from build123d import *

# Parameters (mm, degrees)
SKETCH2_W               = 19.05
SKETCH2_H               = 6.35
BOSS_EXTRUDE1_DEPTH     = 2.54
SKETCH3_W               = 2.54
SKETCH3_H               = 6.35
BOSS_EXTRUDE2_DEPTH     = 17.78
FILLET1_R               = 6.35
SKETCH4_R               = 1.143
CUT_EXTRUDE1_DEPTH      = 27.820764344
CUT_EXTRUDE2_DEPTH      = 27.940768363
CUT_EXTRUDE2_DEPTH_BACK = 27.940768363
SKETCH5_R               = 1.143


with BuildPart() as part:
    # Sketch2 → Boss-Extrude1 (new body)
    with BuildSketch(Plane(origin=(0, 0, 0), x_dir=(1, 0, 0), z_dir=(0, 1, 0))):
        with Locations((9.525, 3.175)):
            Rectangle(SKETCH2_W, SKETCH2_H)
    extrude(amount=BOSS_EXTRUDE1_DEPTH)

    # Sketch3 → Boss-Extrude2 (add)
    with BuildSketch(Plane(origin=(0, 2.54, 0), x_dir=(1, 0, 0), z_dir=(0, 1, 0))):
        with Locations((17.78, 3.175)):
            Rectangle(SKETCH3_W, SKETCH3_H)
    extrude(amount=BOSS_EXTRUDE2_DEPTH)

    # Fillet1
    fillet1_edges = [part.edges().sort_by_distance(p)[0] for p in [
        (16.51, 2.54, -3.175),
    ]]
    fillet(fillet1_edges, radius=FILLET1_R)

    # Sketch4 → Cut-Extrude1 (cut, through all)
    with BuildSketch(Plane(origin=(0, 2.54, 0), x_dir=(1, 0, 0), z_dir=(0, 1, 0))):
        with Locations(Location((6.35, 3.175, 0), (0, 0, 270))):
            Circle(SKETCH4_R)
    extrude(amount=-CUT_EXTRUDE1_DEPTH, mode=Mode.SUBTRACT)

    # Sketch5 → Cut-Extrude2 (cut, two sides: drawn at the far end of the back side and taken through both)
    with BuildSketch(Plane.ZY.offset(-16.51).offset(-CUT_EXTRUDE2_DEPTH_BACK)):
        with Locations((-3.175, 15.24)):
            Circle(SKETCH5_R)
        with Locations((-3.175, 4.826)):
            Circle(SKETCH5_R)
    extrude(amount=CUT_EXTRUDE2_DEPTH + CUT_EXTRUDE2_DEPTH_BACK, mode=Mode.SUBTRACT)


solid = part.part
Source: CAD feature listing. Evaluate the final solid. Frame: model axes, mm. A direction names the side the tool comes from. Round coordinates to 2 decimals unless told otherwise and drop trailing zeros. Loops run counter-clockwise (first coordinate to the right, second up) from the corner with the lowest first, then second, coordinate; pieces in that order, holes last.
Q1. First-contact query: P1, Ø1, axis at x = 14.5, z = -1, coming from the +Y side; P2, Ø1.8, axis at x = 6.35, z = -3.175, coming from the +Y side; P3, Ø1.9, axis at x = 4, z = -3, coming from the +Y side. Flat tips, straight axial feed; report the tip coordinate or a pass-through.
Q2. Section C-C, the plane z = -2.5. Return loops of the section in (x, y).
Q3. Access query for faces 1 (the face through (5, 2.54, -3)), 2 (the face through (7.12, 1.29, -4.02)). Directions: +Z, -Z, +X, -X, +Y, -Y. A direction counts if a zero-diameter tool reaches every point of the face in a straight line with its end or side. Return the directions, or none.
Q4. Ray query, line 1 (Z direction, x = 17.65, y = 15.24); line 2 (Y direction, x = 8.25, z = -4.5); line 3 (X direction, y = 12.25, z = -1.25). Return the intervals inside material, ascending.
Q5. Mould query, pull axis Z, two halves, no side actions, for faces 3 (the face through (0, 1, -3)), 4 (the face through (16, 6, 0)), 5 (the face through (17.04, 3.71, -3.42)), 6 (the face through (17.798, 16.373, -3.324)). Classes: pulls with the +Z half, pulls with the -Z half, needs draft (parallel to the pull), parting line crosses it, or undercut.
Q6. Section A-A, the plane x = 6.35. Return loops of the section in (y, z).
Q7. Section B-B, the plane y = 15.24. Return loops of the section in (x, z), plus the area to 3 significant figures.
Q8. Section D-D, the plane z = -5.5. Return loops of the section in (x, y).
Solutions:
1. P1: stops at y = 4.78
1. P2: passes through
1. P3: stops at y = 2.54
2. outline: (0, 0) - (5.43, 0) - (5.43, 2.54) - (0, 2.54) - close; (7.27, 0) - (19.05, 0) - (19.05, 3.9) - (14.09, 3.9) arc R6.35 cw to (10.16, 2.54) - (7.27, 2.54) - close; (15.68, 5.75) - (19.05, 5.75) - (19.05, 14.32) - (16.51, 14.32) - (16.51, 8.89) arc R6.35 cw to start; (16.51, 16.16) - (19.05, 16.16) - (19.05, 20.32) - (16.51, 20.32) - close
3. face 1: +Z, -Z, -X, +Y
3. face 2: +Y, -Y
4. line 1: z = -6.35 to -4.32, -2.03 to 0
4. line 2: y = 0 to 2.54
4. line 3: x = 16.51 to 19.05
5. face 3: needs draft
5. face 4: pulls with the +Z half
5. face 5: undercut
5. face 6: undercut
6. outline: (0, -6.35) - (2.54, -6.35) - (2.54, -4.32) - (0, -4.32) - close; (0, -2.03) - (2.54, -2.03) - (2.54, 0) - (0, 0) - close
7. outline: (16.51, -6.35) - (19.05, -6.35) - (19.05, -4.32) - (16.51, -4.32) - close; (16.51, -2.03) - (19.05, -2.03) - (19.05, 0) - (16.51, 0) - close
7. area: 10.3 mm2
8. outline: (0, 0) - (19.05, 0) - (19.05, 20.32) - (16.51, 20.32) - (16.51, 8.89) arc R6.35 cw to (10.16, 2.54) - (0, 2.54) - close
